Read the model definition and answer for the solid it produces. Units are mm, in the model's axes. Face numbers are marked on the shaded views. A direction names the side the tool comes from. Give positions to 0.01 mm unless a question says otherwise; leave off trailing zeros. Write each loop counter-clockwise with the first axis right and the second up, starting at its lowest first coordinate (ties: lowest second). Pieces come first, ordered by that corner, then holes. Notation, with made-up numbers: (-32.75, 53) - (-25.75, 53) arc R22 cw to (-25.75, 77) - close; hole circle Ø3 at (8.25, 44.5). An arc over 180 degrees is marked (long way). Answer as CSV lines item,"result".
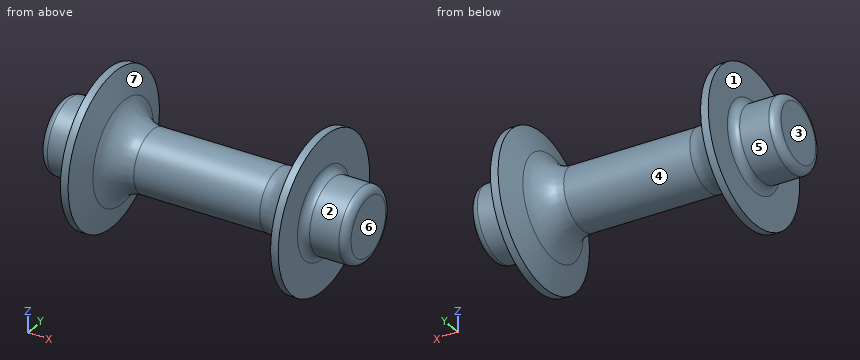
Autodesk Fusion 360 part; units mm, degrees
sketch "Sketch1" plane through (0, 0, 0) normal (0, 1, 0) x (1, 0, 0)
  line L0 (0, 0) -> (10, 0)
  line L1 (10, 0) -> (10, -2.4)
  line L2 (10, -2.4) -> (7.1, -2.4)
  line L3 (7.1, -2.4) -> (7.1, -5)
  line L4 (7.1, -5) -> (6.6, -5)
  line L5 (6.6, -5) -> (5.5081, -2)
  line L6 (5.5081, -2) -> (0, -2)
  line L7 (0, -2) -> (0, 0)
  dimension "d1" = 2.4
  dimension "d6" = 0.5
  dimension "d7" = 2
  dimension "d8" = 5
  dimension "d9" = 2.9
  dimension "d13" = 110
  dimension "d14" = 10
revolve "Revolve1" add sketch "Sketch1" angle 360 about axis through (0, 0, 0) along (1, 0, 0)
mirror "Mirror1" about plane through (0, 0, 0) normal (-1, 0, 0) of bodies 1 merged
fillet "Fillet2" radius 0.5 4 edges at (-7.1, -0.8679, -2.2376) (7.1, -0.8679, -2.2376) (10, -0.8679, -2.2376) (-10, -0.8679, -2.2376)
fillet "Fillet2" radius 2 2 edges at (5.5081, -0.7232, -1.8647) (-5.5081, -0.7232, -1.8647)
(1) A cutting plane is placed at A-A (x = 3.5). Write down the section's boundary in (y, z).
Worked out:
outline,"circle Ø4 at (0, 0)"
(2) Find the intervals of material crossed by L1, parallel to X at y = 0.25, z = -4; L2, parallel to X at y = -3, z = -1.25; L3, parallel to Y at x = 7, z = 3.75, in increasing order.
Worked out:
L1,"x = -7.1 to -6.24, 6.24 to 7.1"
L2,"x = -7.1 to -5.96, 5.96 to 7.1"
L3,"y = -3.31 to 3.31"
(3) For the marked faces 1, 2, 3 and 4, determine the directions among +Z, -Z, +X, -X, +Y, -Y from which every point of the face is accessible in a straight line to the end or side of a thin tool.
Worked out:
face 1,"-X"
face 2,"+X"
face 3,"+Z, -Z, -X, +Y, -Y"
face 4,"none"
(4) Each of these flat-tipped pins is pushed along its axis until it touches: P1, Ø4, axis at x = 0, z = 1.5, coming from the -Y side; P2, Ø2, axis at y = -3, z = 0, coming from the +X side; P3, Ø6, axis at x = -4.5, z = 3, coming from the -Y side. Where does it stop, or does it pass through?
Worked out:
P1,"stops at y = -2"
P2,"stops at x = 9.99"
P3,"stops at y = -4.93"
(5) The mould has two halves that part along X. Classify the marked faces 5, 6 and 7: +X half, -X half, draft (parallel to the pull), parting line (faces both ways), or undercut.
Worked out:
face 5,"draft"
face 6,"+X half"
face 7,"undercut"
(6) A cutting plane is placed at B-B (x = 9.25). Write down the section's boundary in (y, z), and give its area (3 significant figures).
Worked out:
outline,"circle Ø4.8 at (0, 0)"
area,"18.1 mm^2"
